The listing builds one solid part. Answer for the finished solid, in the listing's coordinates (mm). A direction names the side the tool comes from. Coordinates: 2 decimals unless noted, no trailing zeros. Write each loop counter-clockwise with the first axis right and the second up, starting at its lowest first coordinate (ties: lowest second). Pieces come first, ordered by that corner, then holes.
(1) The part is cut by section B-B on z = -88.3. Give the number of separate pieces and of enclosed holes in the cut face, plus the area to 3 significant figures.
(2) Given P1, Ø1.5, axis at x = -13, y = 6.5, coming from the +Z side; P2, Ø10, axis at x = 13, y = 0, coming from the -Z side; P3, Ø5, axis at x = 17, y = 6.5, coming from the +Z side, each flat-ended and moving along its own axis, determine where each tip first touches the part or whether it passes through.
(3) For a pull along X with two mould halves and no side action, classify faces 1 (the flat face through (0, -7, 0)), 2 (the cylindrical face through (14.1, 18.5, -56.1)), 3 (the flat face through (24.376, 17.337, -42.821)), 4 (the cylindrical face through (-24.16, 20.4, -44.23)) as +X half, -X half, draft (parallel to the pull), parting line (faces both ways), or undercut.
(4) The part is cut by section A-A on z = 40. Determine the outline of the cut face in (x, y).
(5) Which of the six approach directions +Z, -Z, +X, -X, +Y, -Y give full straight-line access (tool end or side, diameter ignored) to faces 5 (the flat face through (8, 14, 3)), 6 (the cylindrical face through (31, 12, 3)), 7 (the flat face through (-2, 19, -24)), 8 (the flat face through (-29.736, 0.131, 2.535))?
(6) Straight lines are drawn through the part: line 1 (Y direction, x = 27, z = 1.8); line 2 (Z direction, x = -8, y = -1); line 3 (Y direction, x = 8.5, z = -63). For each, find the intervals that lie inside material, in ascending order.
from build123d import *

# Parameters (mm, degrees)
SKETCH1_W           = 60
SKETCH1_H           = 32
BOSS_EXTRUDE1_DEPTH = 5
SKETCH2_R           = 1.5
CUT_EXTRUDE1_DEPTH  = 5
SKETCH4_R           = 5
CUT_EXTRUDE2_DEPTH  = 5
SKETCH5_W           = 60
SKETCH5_H           = 5
BOSS_EXTRUDE2_DEPTH = 97
SKETCH6_R           = 1.5
CUT_EXTRUDE3_DEPTH  = 100
CUT_EXTRUDE4_DEPTH  = 100
BOSS_EXTRUDE3_DEPTH = 45
SKETCH9_W           = 26
SKETCH9_H           = 23
BOSS_EXTRUDE4_DEPTH = 5
SKETCH10_R          = 5
CUT_EXTRUDE5_DEPTH  = 5
SKETCH17_W          = 16
SKETCH17_H          = 3
CUT_EXTRUDE6_DEPTH  = 10
SKETCH18_R          = 1.5
CUT_EXTRUDE7_DEPTH  = 10
FILLET3_R           = 2
FILLET4_R           = 2
FILLET5_R           = 2
SKETCH34_R          = 4
SKETCH34_R_2        = 1.5
BOSS_EXTRUDE5_DEPTH = 5
SKETCH36_R          = 4
SKETCH36_R_2        = 1.5
BOSS_EXTRUDE6_DEPTH = 5
SKETCH37_R          = 4
SKETCH37_R_2        = 1.5
BOSS_EXTRUDE7_DEPTH = 5
SKETCH38_R          = 4
SKETCH38_R_2        = 1.5
BOSS_EXTRUDE8_DEPTH = 5
SKETCH40_W          = 4
SKETCH40_H          = 39.348212258
CUT_EXTRUDE8_DEPTH  = 10
FILLET6_R           = 1.5
SKETCH43_R          = 1.5
CUT_EXTRUDE10_DEPTH = 9


with BuildPart() as part:
    # Sketch1 → Boss-Extrude1 (new body)
    with BuildSketch(Plane.XY):
        Rectangle(SKETCH1_W, SKETCH1_H)
    extrude(amount=BOSS_EXTRUDE1_DEPTH)

    # Sketch2 → Cut-Extrude1 (cut)
    with BuildSketch(Plane.XY.offset(5)):
        with Locations((27, 12)):
            Circle(SKETCH2_R)
        with Locations((27, -12)):
            Circle(SKETCH2_R)
        with Locations((-27, -12)):
            Circle(SKETCH2_R)
        with Locations((-27, 12)):
            Circle(SKETCH2_R)
    extrude(amount=-CUT_EXTRUDE1_DEPTH, mode=Mode.SUBTRACT)

    # Sketch4 → Cut-Extrude2 (cut)
    with BuildSketch(Plane.XY.offset(5)):
        Circle(SKETCH4_R)
    extrude(amount=-CUT_EXTRUDE2_DEPTH, mode=Mode.SUBTRACT)

    # Sketch5 → Boss-Extrude2 (add)
    with BuildSketch(Plane.XY.offset(5)):
        with Locations((0, 18.5)):
            Rectangle(SKETCH5_W, SKETCH5_H)
    extrude(amount=-BOSS_EXTRUDE2_DEPTH)

    # Sketch6 → Cut-Extrude3 (cut)
    with BuildSketch(Plane.XZ.offset(-16)):
        with Locations(Location((15, -57.3, 0), (0, 0, 270))):
            Circle(SKETCH6_R)
        with Locations(Location((-16, -57.3, 0), (0, 0, 270))):
            Circle(SKETCH6_R)
        with Locations(Location((15, -88.3, 0), (0, 0, 270))):
            Circle(SKETCH6_R)
        with Locations(Location((-16, -88.3, 0), (0, 0, 270))):
            Circle(SKETCH6_R)
    extrude(amount=-CUT_EXTRUDE3_DEPTH, mode=Mode.SUBTRACT)

    # Sketch7 → Cut-Extrude4 (cut)
    with BuildSketch(Plane(origin=(0, 21, 0), x_dir=(1, 0, 0), z_dir=(0, 1, 0))):
        Polygon((30, -5), (18.592432289, 92), (30, 92), align=None)
        Polygon((-30, -5), (-19.627140112, 92), (-30, 92), align=None)
    extrude(amount=-CUT_EXTRUDE4_DEPTH, mode=Mode.SUBTRACT)

    # Sketch8 → Boss-Extrude3 (add)
    with BuildSketch(Plane.XY.offset(5)):
        Polygon((13, 13), (-13, 13), (-13, -10), (-10, -10), (-10, 10), (10, 10), (10, -10), (13, -10), align=None)
    extrude(amount=BOSS_EXTRUDE3_DEPTH)

    # Sketch9 → Boss-Extrude4 (add)
    with BuildSketch(Plane.XY.offset(50)):
        with Locations((0, 1.5)):
            Rectangle(SKETCH9_W, SKETCH9_H)
    extrude(amount=-BOSS_EXTRUDE4_DEPTH)

    # Sketch10 → Cut-Extrude5 (cut)
    with BuildSketch(Plane.XY.offset(50)):
        Circle(SKETCH10_R)
    extrude(amount=-CUT_EXTRUDE5_DEPTH, mode=Mode.SUBTRACT)

    # Sketch17 → Cut-Extrude6 (cut)
    with BuildSketch(Plane.XY.offset(5)):
        with Locations((0, 14.5)):
            Rectangle(SKETCH17_W, SKETCH17_H)
    extrude(amount=-CUT_EXTRUDE6_DEPTH, mode=Mode.SUBTRACT)

    # Sketch18 → Cut-Extrude7 (cut)
    with BuildSketch(Plane(origin=(0, 13, 0), x_dir=(1, 0, 0), z_dir=(0, 1, 0))):
        with Locations(Location((0, -23, 0), (0, 0, 180))):
            Circle(SKETCH18_R)
    extrude(amount=-CUT_EXTRUDE7_DEPTH, mode=Mode.SUBTRACT)

    # Fillet3
    fillet3_edges = [part.edges().sort_by_distance(p)[0] for p in [
        (0, 21, 5),
        (24.296216145, 21, -43.5),
        (-24.813570056, 21, -43.5),
    ]]
    fillet(fillet3_edges, radius=FILLET3_R)

    # Fillet4
    fillet4_edges = [part.edges().sort_by_distance(p)[0] for p in [
        (0, -10, 50),
        (13, 1.5, 50),
        (0, 13, 50),
        (-13, 1.5, 50),
    ]]
    fillet(fillet4_edges, radius=FILLET4_R)

    # Fillet5
    fillet5_edges = [part.edges().sort_by_distance(p)[0] for p in [
        (11.5, -10, 5),
        (13, 1.5, 5),
        (10.5, 13, 5),
        (-13, 1.5, 5),
        (-11.5, -10, 5),
        (-10.5, 13, 5),
    ]]
    fillet(fillet5_edges, radius=FILLET5_R)

    # Sketch34 → Boss-Extrude5 (add)
    with BuildSketch(Plane.XY.offset(5)):
        with Locations((-27, 12)):
            Circle(SKETCH34_R)
        with Locations((-27, 12)):
            Circle(SKETCH34_R_2, mode=Mode.SUBTRACT)
    extrude(amount=-BOSS_EXTRUDE5_DEPTH)

    # Sketch36 → Boss-Extrude6 (add)
    with BuildSketch(Plane.XY.offset(5)):
        with Locations((-27, -12)):
            Circle(SKETCH36_R)
        with Locations((-27, -12)):
            Circle(SKETCH36_R_2, mode=Mode.SUBTRACT)
    extrude(amount=-BOSS_EXTRUDE6_DEPTH)

    # Sketch37 → Boss-Extrude7 (add)
    with BuildSketch(Plane.XY.offset(5)):
        with Locations((27, 12)):
            Circle(SKETCH37_R)
        with Locations((27, 12)):
            Circle(SKETCH37_R_2, mode=Mode.SUBTRACT)
    extrude(amount=-BOSS_EXTRUDE7_DEPTH)

    # Sketch38 → Boss-Extrude8 (add)
    with BuildSketch(Plane.XY.offset(5)):
        with Locations((27, -12)):
            Circle(SKETCH38_R)
        with Locations((27, -12)):
            Circle(SKETCH38_R_2, mode=Mode.SUBTRACT)
    extrude(amount=-BOSS_EXTRUDE8_DEPTH)

    # Sketch40 → Cut-Extrude8 (cut)
    with BuildSketch(Plane(origin=(0, 21, 0), x_dir=(1, 0, 0), z_dir=(0, 1, 0))):
        with Locations((12, 24.674106129)):
            Rectangle(SKETCH40_W, SKETCH40_H)
        with Locations((0, 24.674106129)):
            Rectangle(SKETCH40_W, SKETCH40_H)
        with Locations((-12, 24.674106129)):
            Rectangle(SKETCH40_W, SKETCH40_H)
    extrude(amount=-CUT_EXTRUDE8_DEPTH, mode=Mode.SUBTRACT)

    # Fillet6
    fillet6_edges = [part.edges().sort_by_distance(p)[0] for p in [
        (-10, 18.5, -5),
        (-14, 18.5, -5),
        (-14, 18.5, -44.348212258),
        (-10, 18.5, -44.348212258),
        (2, 18.5, -5),
        (-2, 18.5, -5),
        (-2, 18.5, -44.348212258),
        (2, 18.5, -44.348212258),
        (14, 18.5, -5),
        (10, 18.5, -5),
        (10, 18.5, -44.348212258),
        (14, 18.5, -44.348212258),
    ]]
    fillet(fillet6_edges, radius=FILLET6_R)

    # Sketch43 → Cut-Extrude10 (cut)
    with BuildSketch(Plane.ZY.offset(13)):
        with Locations((40, 1.5)):
            Circle(SKETCH43_R)
    extrude(amount=-CUT_EXTRUDE10_DEPTH, mode=Mode.SUBTRACT)


solid = part.part
Model answer:
1. separate pieces: 3
1. enclosed holes: 0
1. area: 164 mm2
2. P1: stops at z = 49.56
2. P2: stops at z = 0
2. P3: stops at z = 5.06
3. face 1: draft
3. face 2: undercut
3. face 3: +X half
3. face 4: -X half
4. outline: (-13, -10) - (-10, -10) - (-10, 0) - (-13, 0) - close; (-13, 3) - (-10, 3) - (-10, 10) - (10, 10) - (10, -10) - (13, -10) - (13, 13) - (-13, 13) - close
5. face 5: +Z, -Z
5. face 6: -Z, +X
5. face 7: +Y, -Y
5. face 8: -Z, -X
6. line 1: y = -16 to -13.5, -10.5 to 10.5, 13.5 to 21
6. line 2: z = 0 to 5, 45 to 50
6. line 3: y = 16 to 21
